from build123d import *

# Parameters (mm, degrees)
F1_DEPTH = 1
F2_R     = 5
F3_R     = 2
F4_R     = 10
F6_DEPTH = 1
F8_R     = 5


with BuildPart() as f1:
    # F0 (on Right) → F1 (new body)
    with BuildSketch(Plane.YZ):
        Polygon((90, 0), (120, 0), (0, 84.8264595052), (-120, 0), (-90, 0), (-90, -20), (90, -20), align=None)
    extrude(amount=F1_DEPTH)

    # F2
    f2_edges = [f1.edges().sort_by_distance(p)[0] for p in [
        (0.5, -90, -20),
        (0.5, 90, -20),
    ]]
    fillet(f2_edges, radius=F2_R)

    # F3
    f3_edges = [f1.edges().sort_by_distance(p)[0] for p in [
        (0.5, 120, 0),
        (0.5, -120, 0),
    ]]
    fillet(f3_edges, radius=F3_R)

    # F4
    f4_edges = [f1.edges().sort_by_distance(p)[0] for p in [
        (0.5, 0, 84.82646),
    ]]
    fillet(f4_edges, radius=F4_R)

    # F5 (on face) → F6 (join, through all)
    with BuildSketch(Plane.YZ.offset(1)):
        with BuildLine():
            Line((-30.2697404192, 63.4291685894), (-22.1039292974, 69.2014756431))
            Line((-22.1039292974, 69.2014756431), (-27.8762363511, 77.3672867649))
            ThreePointArc((-27.8762363511, 77.3672867649), (-34.8452954389, 78.564038799), (-36.042047473, 71.5949797112))
            Line((-36.042047473, 71.5949797112), (-30.2697404192, 63.4291685894))
        make_face()
    extrude(amount=-F6_DEPTH)

    # F7: F1 across plane


with BuildPart() as f1_1:
    add(f1.part)
    add(f1.part.mirror(Plane.XZ))

    # F8
    f8_edges = [f1_1.edges().sort_by_distance(p)[0] for p in [
        (0.5, -30.26974, 63.429169),
        (0.5, -22.103929, 69.201476),
        (0.5, 22.103929, 69.201476),
        (0.5, 30.26974, 63.429169),
    ]]
    fillet(f8_edges, radius=F8_R)


solid = f1_1.part
Check sheet for the modelled part. Datum: model origin and axes. Units: mm. A direction names the side the tool comes from. Round coordinates to 2 decimals unless told otherwise and drop trailing zeros. Order: outer loops, then holes, each group sorted by start corner. A loop starts at its lowest first (then second) coordinate and runs counter-clockwise, first axis right, second up. Notation, with made-up numbers: M 8,51 L 29,51 A24 cw 29,81 Z; hole C 49.5,87.5 d2. An arc over 180 degrees is marked long. One line per item, written item: value. Start each with the question number.
1. Section check B-B on y = -95. Enter the section's corners in (x, z).
2. Access from +Z, -Z, +X, -X, +Y, -Y to the whole of each face (thin tool, end or side, straight path). Record for faces 1 (the cylindrical face through (0.51, -34.75, 78.63)), 2 (the flat face through (0.49, -11.81, 76.48)).
3. Scan lines: line 1 along Y through (x, z) = (0.9, 78); line 2 along Z through (x, y) = (0.55, -25); line 3 along Y through (x, z) = (0.55, 8). Record each from-to range of solid material in increasing order.
4. Section check A-A on x = 0.45. Enter the section's corners in (y, z), and give its area (3 significant figures).
5. Section check C-C on z = 42. Enter the section's corners in (x, y).
Results found:
1. outline: M 0,0 L 1,0 L 1,17.67 L 0,17.67 Z
2. face 1: +X, -X
2. face 2: +Z, +X, -X
3. line 1: -35.51 to -28.41, -9.66 to 9.66, 28.41 to 35.51
3. line 2: -20 to 73.3
3. line 3: -108.68 to 108.68
4. outline: M -114.86,3.63 A2 ccw -113.71,0 L -90,0 L -90,-15 A5 ccw -85,-20 L 85,-20 A5 ccw 90,-15 L 90,0 L 113.71,0 A2 ccw 114.86,3.63 L 34.35,60.54 A5 cw 33.16,67.51 L 36.04,71.59 A5 ccw 27.88,77.37 L 24.99,73.28 A5 cw 18.02,72.09 L 5.77,80.75 A10 ccw -5.77,80.75 L -18.02,72.09 A5 cw -24.99,73.28 L -27.88,77.37 A5 ccw -36.04,71.59 L -33.16,67.51 A5 cw -34.35,60.54 Z
4. area: 14,000 mm^2
5. outline: M 0,-60.58 L 1,-60.58 L 1,60.58 L 0,60.58 Z
